from build123d import *

# Parameters (mm, degrees)
SKETCH1_W                 = 24.765
SKETCH1_H                 = 12.7
BOSS_EXTRUDE1_DEPTH       = 9.525
CUT_EXTRUDE1_DEPTH        = 10.525
FILLET1_R                 = 5.08
F_6_32_TAPPED_HOLE2_D     = 2.7051
F_6_32_TAPPED_HOLE1_D     = 2.7051
F_6_32_TAPPED_HOLE1_DEPTH = 11.176


with BuildPart() as part:
    # Sketch1 → Boss-Extrude1 (new body)
    with BuildSketch(Plane.XY):
        Rectangle(SKETCH1_W, SKETCH1_H)
    extrude(amount=BOSS_EXTRUDE1_DEPTH)

    # Sketch2 → Cut-Extrude1 (cut, through all)
    with BuildSketch(Plane.XY.offset(9.525)):
        Polygon((4.7625, 4.7625), (-4.7625, 4.7625), (-4.7625, -4.7625), (4.7625, -4.7625), (4.7625, -3.175), (-3.175, -3.175), (-3.175, 3.175), (4.7625, 3.175), align=None)
    extrude(amount=-CUT_EXTRUDE1_DEPTH, mode=Mode.SUBTRACT)

    # Fillet1
    fillet1_edges = [part.edges().sort_by_distance(p)[0] for p in [
        (-12.3825, 6.35, 4.7625),
        (12.3825, 6.35, 4.7625),
        (12.3825, -6.35, 4.7625),
        (-12.3825, -6.35, 4.7625),
    ]]
    fillet(fillet1_edges, radius=FILLET1_R)

    # #6-32 Tapped Hole2 (through all)
    with Locations(Plane.XY.offset(9.525)):
        with Locations((-8.89, 0), (8.89, 0)):
            Hole(F_6_32_TAPPED_HOLE2_D / 2)

    # #6-32 Tapped Hole1
    with Locations(Plane(origin=(0, 6.35, 0), x_dir=(1, 0, 0), z_dir=(0, 1, 0))):
        with Locations((0, -4.7625)):
            Hole(F_6_32_TAPPED_HOLE1_D / 2, depth=F_6_32_TAPPED_HOLE1_DEPTH)


solid = part.part
Model file for the job. Use its own axes, mm. A direction names the side the tool comes from. Give positions to 0.01 mm unless a question says otherwise; leave off trailing zeros. Write each loop counter-clockwise with the first axis right and the second up, starting at its lowest first coordinate (ties: lowest second). Pieces come first, ordered by that corner, then holes. Notation, with made-up numbers: M -22,40 L 30,40 A25 cw 30,73 Z; hole C -13,4 d9. An arc over 180 degrees is marked long. One line per item, written item: value. Start each with the question number.
Q1. Two-plate mould, pull along Z, no slides. Class faces 1 (the flat face through (0, -6.35, 5)), 2 (the flat face through (0, -4.826, 5)), 3 (the flat face through (0, 0, 9.525)), 4 (the cylindrical face through (0.18, 5.55, 3.42)): +Z half, -Z half, draft (parallel to the pull), parting line (faces both ways), or undercut.
Q2. 3-axis set-ups, long thin cutter, end or side, ignore diameter. For faces 5 (the flat face through (-4.762, 0, 5)), 6 (the cylindrical face through (-10.934, 4.822, 4.829)): which of +Z, -Z, +X, -X, +Y, -Y reach the whole face in a straight line?
Q3. Saw through at B-B, the plane y = 0. Write the cut outline in (x, z) (1 decimal), plus the area to 3 significant figures.
Q4. Probe probe 1 along X at (y, z) = (1.5, 6.75) (1 decimal); probe 2 along Z at (x, y) = (0, 1.25) (3 decimals); probe 3 along X at (y, z) = (-1, 5.75) (1 decimal). List the from-to ranges inside material, lowest first. Write a range as [from, to].
Q5. Saw through at A-A, the plane x = 0. State how many separate pieces and enclosed holes the cut face has, plus the area to 3 significant figures.
Q6. Drop flat-ended pins along their axis: pin 1 Ø0.8 at (y, z) = (4, 3.5) entering from -X; pin 2 Ø1.7 at (y, z) = (-4, 6.5) entering from -X; pin 3 Ø2 at (x, z) = (0, 4.5) entering from +Y; pin 4 Ø2.5 at (x, y) = (8.89, 0) entering from -Z (3 decimals). Give the stop position or say it passes through.
Output values:
1. face 1: draft
1. face 2: undercut
1. face 3: +Z half
1. face 4: undercut
2. face 5: +Z, -Z
2. face 6: +Z, -Z, -X, +Y
3. outline: M -12.4,0 L -10.2,0 L -10.2,9.5 L -12.4,9.5 Z; M -7.5,0 L -4.8,0 L -4.8,9.5 L -7.5,9.5 Z; M -3.2,0 L 7.5,0 L 7.5,9.5 L -3.2,9.5 Z; M 10.2,0 L 12.4,0 L 12.4,9.5 L 10.2,9.5 Z; hole C 0,4.8 d2.7
3. area: 163 mm²
4. probe 1: x = [-12.4, -4.8], [-3.2, 12.4]
4. probe 2: z = [0, 3.41], [6.115, 9.525]
4. probe 3: x = [-12.4, -9.8], [-8, -4.8], [-3.2, -0.9], [0.9, 8], [9.8, 12.4]
5. separate pieces: 5
5. enclosed holes: 0
5. area: 69.1 mm²
6. pin 1: stops at x = -11.82
6. pin 2: stops at x = -12.02
6. pin 3: stops at y = -4.83
6. pin 4: passes through
